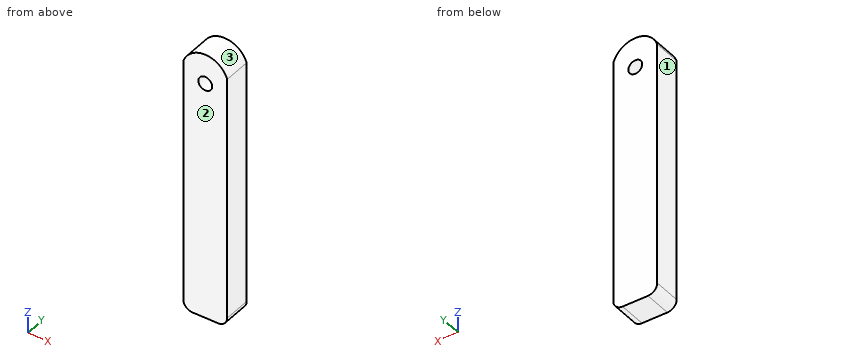
from build123d import *

# Parameters (mm, degrees)
ESQUISSE1_R        = 1.5
BOSS_EXTRU_1_DEPTH = 6
CONG_1_R           = 2


with BuildPart() as part:
    # Esquisse1 → Boss.-Extru.1 (new body)
    with BuildSketch(Plane(origin=(0, 0, 0), x_dir=(1, 0, 0), z_dir=(0, 1, 0))):
        with BuildLine():
            Line((4.75, 40), (-4.75, 40))
            Line((-4.75, 40), (-4.75, -15))
            ThreePointArc((-4.75, -15), (0, -18.4387505), (4.75, -15))
            Line((4.75, -15), (4.75, 40))
        make_face()
        with Locations((0, -12)):
            Circle(ESQUISSE1_R, mode=Mode.SUBTRACT)
    extrude(amount=BOSS_EXTRU_1_DEPTH)

    # Congé1
    cong_1_edges = [part.edges().sort_by_distance(p)[0] for p in [
        (-4.75, 3, -40),
        (4.75, 3, -40),
    ]]
    fillet(cong_1_edges, radius=CONG_1_R)


solid = part.part
Model file for the job. Use its own axes, mm. Face numbers are marked on the shaded views. Give positions to 0.01 mm unless a question says otherwise; leave off trailing zeros. Order: outer loops, then holes, each group sorted by start corner. A loop starts at its lowest first (then second) coordinate and runs counter-clockwise, first axis right, second up. Notation, with made-up numbers: M 63,78.5 L 105,78.5 A12 cw 105,95.5 Z; hole C 67,9.25 d9. An arc over 180 degrees is marked long. Put each result on its own line as item: value. Start each with the question number.
(1) Pull direction X, two halves, no side cores. Call the marked faces 1, 2 and 3: released by +X, released by -X, zero draft, split by the parting line, or undercut.
(2) Band-saw the part on A-A on z = 12. Give the cut face in (x, y).
(3) Band-saw the part on C-C on x = 0. Give the cut face in (y, z), then the cut area to 3 significant figures.
(4) Band-saw the part on B-B on y = 0.7. Give the cut face in (x, z), then the cut area to 3 significant figures.
(5) Drill centre lines: L1, parallel to X at y = 3.3, z = 12; L2, parallel to Z at x = 0, y = 3.85; L3, parallel to Z at x = 4.25, y = 2.45. Where is each one in solid material? Low to high. Write a range as [from, to].
(6) Band-saw the part on D-D on x = 4.25. Give the cut face in (y, z).
Results below:
1. face 1: released by -X
1. face 2: zero draft
1. face 3: split by the parting line
2. outline: M -4.75,0 L -1.5,0 L -1.5,6 L -4.75,6 Z; M 1.5,0 L 4.75,0 L 4.75,6 L 1.5,6 Z
3. outline: M 0,-40 L 6,-40 L 6,10.5 L 0,10.5 Z; M 0,13.5 L 6,13.5 L 6,18.44 L 0,18.44 Z
3. area: 333 mm2
4. outline: M -4.75,-38 A2 ccw -2.75,-40 L 2.75,-40 A2 ccw 4.75,-38 L 4.75,15 A5 ccw -4.75,15 Z; hole C 0,12 d3
4. area: 538 mm2
5. L1: x = [-4.75, -1.5], [1.5, 4.75]
5. L2: z = [-40, 10.5], [13.5, 18.44]
5. L3: z = [-39.32, 16.07]
6. outline: M 0,-39.32 L 6,-39.32 L 6,16.07 L 0,16.07 Z
